The drawing under review shows one solid part. Ordinate dimensions are in mm from its lowest x, y, z. A direction names the side the tool comes from. Round coordinates to 2 decimals unless told otherwise and drop trailing zeros. Order: outer loops, then holes, each group sorted by start corner. A loop starts at its lowest first (then second) coordinate and runs counter-clockwise, first axis right, second up.
1) Consider section D-D (x = 8.25). Give the boundary of the cut face in (y, z).
2) Machinability: for the marked faces 1, 2 and 3, which of the approach directions +Z, -Z, +X, -X, +Y, -Y give a long, thin tool a straight path to every point of the face, cutting with its end or side? Answer none if there is none.
3) Consider section A-A (x = 5). Give the boundary of the cut face in (y, z).
4) Consider section C-C (z = 4.55). Give the boundary of the cut face in (x, y).
5) Consider section B-B (y = 5). Give the boundary of the cut face in (x, z).
6) To check wall thickness, follow L1, parallel to Z at x = 9, y = 8.25; L2, parallel to Y at x = 1.5, z = 1.95; L3, parallel to Z at x = 8, y = 24.5. State the ranges of each line that lie inside material, in increasing order.
7) Clearance check with flat-ended pins moving along their axes: P1, Ø3, axis at x = 3, y = 22, coming from the +Z side; P2, Ø1, axis at y = 7, z = 4, coming from the +X side; P3, Ø0.5, axis at x = 4.5, z = 3, coming from the -Y side; P4, Ø1.5, axis at y = 4.5, z = 2, coming from the +X side. State where each tip first meets the part, or that it passes through.
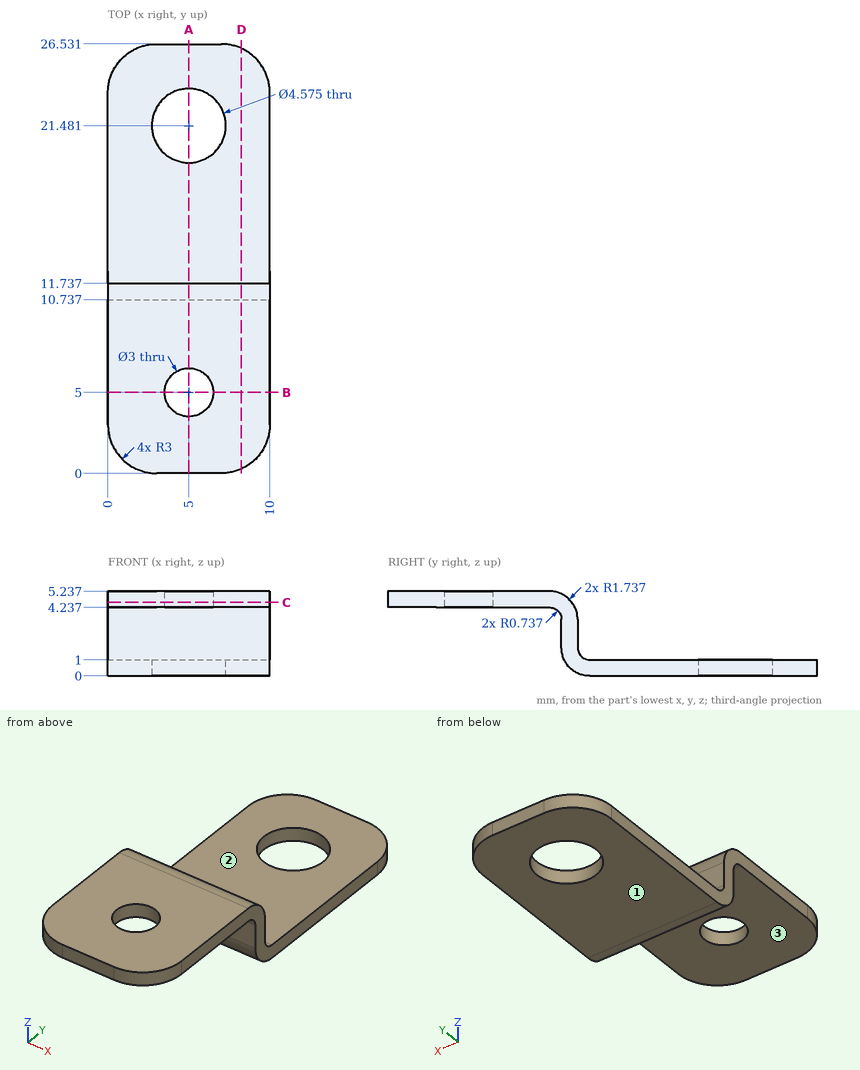
Answer below:
1. outline: (0.27, 4.24) - (10, 4.24) arc R0.74 cw to (10.74, 3.5) - (10.74, 1.74) arc R1.74 ccw to (12.47, 0) - (26.26, 0) - (26.26, 1) - (12.47, 1) arc R0.74 cw to (11.74, 1.74) - (11.74, 3.5) arc R1.74 ccw to (10, 5.24) - (0.27, 5.24) - close
2. face 1: -Z, +X, -X, +Y, -Y
2. face 2: +Z, +X, -X, +Y
2. face 3: -Z, +X, -X, -Y
3. outline: (0, 4.24) - (3.5, 4.24) - (3.5, 5.24) - (0, 5.24) - close; (6.5, 4.24) - (10, 4.24) arc R0.74 cw to (10.74, 3.5) - (10.74, 1.74) arc R1.74 ccw to (12.47, 0) - (19.19, 0) - (19.19, 1) - (12.47, 1) arc R0.74 cw to (11.74, 1.74) - (11.74, 3.5) arc R1.74 ccw to (10, 5.24) - (6.5, 5.24) - close; (23.77, 0) - (26.53, 0) - (26.53, 1) - (23.77, 1) - close
4. outline: (0, 3) arc R3 ccw to (3, 0) - (7, 0) arc R3 ccw to (10, 3) - (10, 11.38) - (0, 11.38) - close; hole circle Ø3 at (5, 5)
5. outline: (0, 4.24) - (3.5, 4.24) - (3.5, 5.24) - (0, 5.24) - close; (6.5, 4.24) - (10, 4.24) - (10, 5.24) - (6.5, 5.24) - close
6. L1: z = 4.24 to 5.24
6. L2: y = 10.74 to 11.74
6. L3: z = 0 to 1
7. P1: stops at z = 1
7. P2: stops at x = 10
7. P3: stops at y = 10.74
7. P4: passes through
